```python
from build123d import *

# Parameters (mm, degrees)
F0_W     = 200
F0_H     = 175
F0_R     = 4.1
F0_R_2   = 2
F1_DEPTH = 6


with BuildPart() as f1:
    # F0 (on Top) → F1 (new body)
    with BuildSketch(Plane.XY):
        Rectangle(F0_W, F0_H)
        with Locations((-84, -57)):
            Circle(F0_R, mode=Mode.SUBTRACT)
        with Locations((-60, -57)):
            Circle(F0_R_2, mode=Mode.SUBTRACT)
        with Locations((-60, -19)):
            Circle(F0_R_2, mode=Mode.SUBTRACT)
        with Locations((0, -57)):
            Circle(F0_R_2, mode=Mode.SUBTRACT)
        with Locations((60, -57)):
            Circle(F0_R_2, mode=Mode.SUBTRACT)
        with Locations((84, -57)):
            Circle(F0_R, mode=Mode.SUBTRACT)
        with Locations((0, -19)):
            Circle(F0_R_2, mode=Mode.SUBTRACT)
        with Locations((60, -19)):
            Circle(F0_R_2, mode=Mode.SUBTRACT)
        with Locations((-60, 19)):
            Circle(F0_R_2, mode=Mode.SUBTRACT)
        with Locations((-84, 57)):
            Circle(F0_R, mode=Mode.SUBTRACT)
        with Locations((-60, 57)):
            Circle(F0_R_2, mode=Mode.SUBTRACT)
        with Locations((0, 19)):
            Circle(F0_R_2, mode=Mode.SUBTRACT)
        with Locations((60, 19)):
            Circle(F0_R_2, mode=Mode.SUBTRACT)
        with Locations((0, 57)):
            Circle(F0_R_2, mode=Mode.SUBTRACT)
        with Locations((60, 57)):
            Circle(F0_R_2, mode=Mode.SUBTRACT)
        with Locations((84, 57)):
            Circle(F0_R, mode=Mode.SUBTRACT)
    extrude(amount=F1_DEPTH)


solid = f1.part
```
Read the model definition and answer for the solid it produces. Units are mm, in the model's axes. Coordinates: 2 decimals unless noted, no trailing zeros. Answer as a JSON object with one key per item and string values.
Q1. A flat-ended cylindrical pin translates along its axis: pin 1 Ø2.5 at (x, y) = (60, 19) entering from -Z. Find the tip coordinate at first contact, or state that the pin passes through.
The answers:
{"pin 1": "passes through"}
Q2. Consider line 1 (Y direction, x = 84, z = 3.95); line 2 (X direction, y = 18, z = 2.1); line 3 (X direction, y = -54.5, z = 4.25). Determine where each line is inside the solid, lowest interval first. Write a range as [from, to].
The answers:
{"line 1": "y = [-87.5, -61.1], [-52.9, 52.9], [61.1, 87.5]", "line 2": "x = [-100, -61.73], [-58.27, -1.73], [1.73, 58.27], [61.73, 100]", "line 3": "x = [-100, -87.25], [-80.75, 80.75], [87.25, 100]"}
Q3. Determine the mould class of faces 1 (the cylindrical face through (-58.092, 19.601, 2.958)), 2 (the flat face through (-1, 1, 6)), 3 (the flat face through (-1, 87.5, 3)) for opening direction Y: pulls with the +Y half, pulls with the -Y half, needs draft (parallel to the pull), parting line crosses it, or undercut.
The answers:
{"face 1": "undercut", "face 2": "needs draft", "face 3": "pulls with the +Y half"}
